Read the model definition and answer for the solid it produces. Units are mm, in the model's axes. A direction names the side the tool comes from. Coordinates: 2 decimals unless noted, no trailing zeros. Write each loop counter-clockwise with the first axis right and the second up, starting at its lowest first coordinate (ties: lowest second). Pieces come first, ordered by that corner, then holes.
(1) Which of the six approach directions +Z, -Z, +X, -X, +Y, -Y give full straight-line access (tool end or side, diameter ignored) to faces 1 (the cylindrical face through (-0.62, 36.463, 37.954)), 2 (the cylindrical face through (-21.73, 28.28, 42.88)), 3 (the flat face through (23.193, 1, 37)), 4 (the flat face through (-25.188, 32.804, 0.428))?
(2) Determine the mould class of faces 5 (the conical face through (1.578, 36.753, 50.629)), 6 (the cylindrical face through (1.465, 28.925, 42.884)), 7 (the flat face through (18.367, 1, 40)), 8 (the flat face through (0, 32, 30.559)) for opening direction Y: pulls with the +Y half, pulls with the -Y half, needs draft (parallel to the pull), parting line crosses it, or undercut.
(3) Given pin 1 (1.5 mm diameter, centred on x = -14, z = -10.5, fed in from +Y); pin 2 (3 mm diameter, centred on x = 9, y = 0.5, fed in from +Z); pin 3 (7 mm diameter, centred on x = 14.5, z = 35, fed in from +Y), each flat-ended and moving along its own axis, determine where each tip first touches the part or whether it passes through.
(4) The part is cut by section D-D, the plane z = -16.5. Determine the outline of the cut face in (x, y), and give its area (3 significant figures).
(5) The part is cut by section A-A, the plane z = 41. State how many separate pieces and enclosed holes the cut face has, and give its area (3 significant figures).
(6) The part is cut by section C-C, the plane y = 7. Determine the outline of the cut face in (x, z).
(7) Straight lines are drawn through the part: line 1 along Y through (x, z) = (0, 38); line 2 along Z through (x, y) = (8.5, 4.5); line 3 along Y through (x, z) = (-2, 37.5). For each, find the intervals that lie inside material, in ascending order.
```python
from build123d import *

# Parameters (mm, degrees)
SKETCH1_W          = 61.11875
SKETCH1_H          = 61.11875
EXTRUDE1_DEPTH     = 36.5125
SKETCH3_OUTSIDE_W  = 81.884
SKETCH3_OUTSIDE_H  = 57.278
CUT_EXTRUDE7_DEPTH = 62
SKETCH4_OUTSIDE_W  = 81.884
SKETCH4_OUTSIDE_H  = 57.278
CUT_EXTRUDE8_DEPTH = 250
SKETCH2_R          = 4.7625
SKETCH2_R_2        = 3.175
EXTRUDE2_DEPTH     = 25
SKETCH5_R          = 4.7625
SKETCH5_R_2        = 3.175
EXTRUDE3_DEPTH     = 25
EXTRUDE4_DEPTH     = 2.54
SKETCH7_R          = 5.76
SKETCH7_R_2        = 4.7625
EXTRUDE5_DEPTH     = 10


with BuildPart() as part:
    # Sketch1 → Extrude1 (new body)
    with BuildSketch(Plane(origin=(0, 0, 0), x_dir=(1, 0, 0), z_dir=(0, 1, 0))):
        Rectangle(SKETCH1_W, SKETCH1_H)
    extrude(amount=EXTRUDE1_DEPTH)

    # Sketch3 outside → Cut-Extrude7 (cut)
    with BuildSketch(Plane.XY.offset(30.559375)):
        with Locations((0, 18.256)):
            Rectangle(SKETCH3_OUTSIDE_W, SKETCH3_OUTSIDE_H)
        Polygon((19.664807265, 36.5125), (30.559375, 29.197130008), (30.559375, 0), (-30.559375, 0), (-30.559375, 29.197130008), (-19.664807265, 36.5125), align=None, mode=Mode.SUBTRACT)
    extrude(amount=-CUT_EXTRUDE7_DEPTH, mode=Mode.SUBTRACT)

    # Sketch4 outside → Cut-Extrude8 (cut)
    with BuildSketch(Plane(origin=(30.559375, 0, 0), x_dir=(0, 0, -1), z_dir=(1, 0, 0))):
        with Locations((0, 18.256)):
            Rectangle(SKETCH4_OUTSIDE_W, SKETCH4_OUTSIDE_H)
        Polygon((-30.559375, 36.5125), (17.867202311, 36.5125), (30.559375, 29.197130008), (30.559375, 0), (-30.559375, 0), align=None, mode=Mode.SUBTRACT)
    extrude(amount=-CUT_EXTRUDE8_DEPTH, mode=Mode.SUBTRACT)

    # Sketch2 → Extrude2 (add)
    with BuildSketch(Plane.XY.offset(30.559375)):
        with Locations((0, 31.741283107)):
            Circle(SKETCH2_R)
        with Locations((0, 31.741283107)):
            Circle(SKETCH2_R_2, mode=Mode.SUBTRACT)
    extrude(amount=EXTRUDE2_DEPTH)

    # Sketch5 → Extrude3 (add)
    with BuildSketch(Plane.XY.offset(30.559375)):
        with Locations((-18.559375, 28.142983961)):
            Circle(SKETCH5_R)
        with Locations((-18.559375, 28.142983961)):
            Circle(SKETCH5_R_2, mode=Mode.SUBTRACT)
    extrude(amount=EXTRUDE3_DEPTH)

    # Sketch6 → Extrude4 (add)
    with BuildSketch(Plane.XZ):
        with BuildLine():
            Line((7.191375, 30.559375), (23.193375, 30.559375))
            Line((23.193375, 30.559375), (23.193375, 44.116625))
            Line((23.193375, 44.116625), (18.367375, 44.116625))
            Line((18.367375, 44.116625), (18.367375, 35.564523256))
            ThreePointArc((18.367375, 35.564523256), (15.192375, 32.389523256), (12.017375, 35.564523256))
            Line((12.017375, 35.564523256), (12.017375, 44.116625))
            Line((12.017375, 44.116625), (7.191375, 44.116625))
            Line((7.191375, 44.116625), (7.191375, 30.559375))
        make_face()
    extrude(amount=-EXTRUDE4_DEPTH)

    # Sketch7 → Extrude5 (add)
    with BuildSketch(Plane.XY.offset(55.559375)):
        with Locations((0, 31.741283107)):
            Circle(SKETCH7_R)
        with Locations((0, 31.741283107)):
            Circle(SKETCH7_R_2, mode=Mode.SUBTRACT)
    extrude(amount=-EXTRUDE5_DEPTH)

    # Sketch8 → Cut-Revolve2 (revolve, cut)
    with BuildSketch(Plane(origin=(0, 0, 0), x_dir=(0, 0, -1), z_dir=(1, 0, 0))):
        Polygon((-55.559375, 36.503783107), (-55.559375, 37.501283107), (-45.559375, 37.501283107), align=None)
    revolve(axis=Axis((0, 31.741283107, 55.559375), (0, 0, -1)), mode=Mode.SUBTRACT)

    # Sketch10 → Revolve1 (revolve)
    with BuildSketch(Plane(origin=(-18.559375, 0, 0), x_dir=(0, 0, -1), z_dir=(1, 0, 0))):
        Polygon((-55.559375, 32.905483961), (-45.559375, 32.905483961), (-45.559375, 33.905483961), align=None)
    revolve(axis=Axis((-18.559375, 28.142983961, 55.559375), (0, 0, -1)))


solid = part.part
```
Computed:
1. face 1: none
1. face 2: +Z
1. face 3: +Z, +X, +Y, -Y
1. face 4: +Z, -Z, -X, +Y
2. face 5: parting line crosses it
2. face 6: undercut
2. face 7: needs draft
2. face 8: undercut
3. pin 1: stops at y = 36.51
3. pin 2: stops at z = 44.12
3. pin 3: stops at y = 2.54
4. outline: (-30.56, 0) - (30.56, 0) - (30.56, 29.2) - (19.66, 36.51) - (-19.66, 36.51) - (-30.56, 29.2) - close
4. area: 2,150 mm2
5. separate pieces: 4
5. enclosed holes: 2
5. area: 104 mm2
6. outline: (-30.56, -30.56) - (30.56, -30.56) - (30.56, 30.56) - (-30.56, 30.56) - close
7. line 1: y = 26.98 to 28.57, 34.92 to 36.5
7. line 2: z = -30.56 to 30.56
7. line 3: y = 27.42 to 29.28, 34.21 to 36.06
